from build123d import *

# Parameters (mm, degrees)
SKETCH5_R                   = 7.5
CUT_EXTRUDE1_DEPTH          = 90
SKETCH6_R                   = 3.5
CUT_EXTRUDE2_DEPTH          = 20
CIRPATTERN1_COUNT           = 6
SKETCH11_R                  = 3.18
CUT_EXTRUDE4_DEPTH          = 101.105860558
SKETCH23_R                  = 30.48
CUT_EXTRUDE6_DEPTH          = 80.122584091
F_1_4_CLEARANCE_HOLE1_D     = 6.5278
F_1_4_CLEARANCE_HOLE1_DEPTH = 15.4203
F_1_4_CLEARANCE_HOLE1_TIP   = 1.961148974
CHAMFER1_SIZE               = 3.175


with BuildPart() as part:
    # Sketch1 → Revolve1 (revolve)
    with BuildSketch(Plane(origin=(0, 0, 0), x_dir=(0, 0, -1), z_dir=(1, 0, 0))):
        Polygon((0, 30.35), (12.7, 30.35), (12.7, 6.35), (30.48, 6.35), (30.48, 0), (15.68, 0), (10.16, -20.600920458), (10.16, -60), (0, -60), align=None)
    revolve(axis=Axis((0, 0, 0), (0, 1, 0)))

    # Sketch5 → Cut-Extrude1 (cut)
    with BuildSketch(Plane.XZ.offset(60)):
        with Locations(Location((0, 0, 0), (0, 0, 270))):
            Circle(SKETCH5_R)
    extrude(amount=-CUT_EXTRUDE1_DEPTH, mode=Mode.SUBTRACT)

    # Sketch6 → Cut-Extrude2 (cut, symmetric)
    with BuildSketch(Plane.XY):
        with Locations((0, 16.659966967)):
            Circle(SKETCH6_R)
    cut_extrude2 = extrude(amount=CUT_EXTRUDE2_DEPTH, both=True, mode=Mode.SUBTRACT)

    # CirPattern1: Cut-Extrude2 ×6 about axis
    cirpattern1_axis = Axis((0, 30.35, 0), (0, -1, 0))
    for i in range(1, CIRPATTERN1_COUNT):
        add(cut_extrude2.rotate(cirpattern1_axis, i * 360 / CIRPATTERN1_COUNT), mode=Mode.SUBTRACT)

    # Sketch11 → Cut-Extrude4 (cut, through all)
    with BuildSketch(Plane(origin=(0, 30.35, 0), x_dir=(1, 0, 0), z_dir=(0, 1, 0))):
        with Locations(Location((0, 0, 0), (0, 0, 270))):
            Circle(SKETCH11_R)
    extrude(amount=-CUT_EXTRUDE4_DEPTH, mode=Mode.SUBTRACT)

    # Sketch23 → Cut-Extrude6 (cut, through all)
    with BuildSketch(Plane(origin=(0, 6.35, 0), x_dir=(1, 0, 0), z_dir=(0, 1, 0))):
        with Locations(Location((0, 0, 0), (0, 0, 90))):
            Circle(SKETCH23_R)
    extrude(amount=CUT_EXTRUDE6_DEPTH, mode=Mode.SUBTRACT)

    # 1_4 Clearance Hole1
    with Locations(Plane(origin=(0, 6.35, 0), x_dir=(1, 0, 0), z_dir=(0, 1, 0))):
        with Locations((3.330049479, 25.294237026), (-20.240427094, 15.531025958), (23.570476573, 9.763211068), (20.240427094, -15.531025958), (-3.330049479, -25.294237026), (-23.570476573, -9.763211068)):
            Hole(F_1_4_CLEARANCE_HOLE1_D / 2, depth=F_1_4_CLEARANCE_HOLE1_DEPTH)
            with Locations((0, 0, -(F_1_4_CLEARANCE_HOLE1_DEPTH + F_1_4_CLEARANCE_HOLE1_TIP / 2))):  # 118° drill point
                Cone(0, F_1_4_CLEARANCE_HOLE1_D / 2, F_1_4_CLEARANCE_HOLE1_TIP, mode=Mode.SUBTRACT)

    # Chamfer1
    chamfer1_edges = [part.edges().sort_by_distance(p)[0] for p in [
        (0, 6.35, 7.5),
    ]]
    chamfer(chamfer1_edges, length=CHAMFER1_SIZE)


solid = part.part
Part model, mm, in its own coordinate system. A direction names the side the tool comes from. Give positions to 0.01 mm unless a question says otherwise; leave off trailing zeros. Loops run counter-clockwise (first coordinate to the right, second up) from the corner with the lowest first, then second, coordinate; pieces in that order, holes last. Notation, with made-up numbers: M -33,-21.75 L -6,-21.75 A24 ccw -6,5.25 Z; hole C 84.25,-38.75 d11. An arc over 180 degrees is marked long. Put each result on its own line as item: value. Start each with the question number.
1) Flat gauge pins, fed straight in: pin 1 (5 mm diameter, centred on y = -5.5, z = 2, fed in from +X); pin 2 (1 mm diameter, centred on y = -46, z = 3, fed in from -X); pin 3 (10 mm diameter, centred on x = -1, y = -33, fed in from +Z); pin 4 (5 mm diameter, centred on x = -20.24, z = -15.53, fed in from +Y). Where does each tip first touch, or does it go through?
2) Saw through at C-C (z = -23.5). List the corners of the cut face in (x, y), then the cut area to 3 significant figures.
3) Saw through at B-B (y = -30). List the corners of the cut face in (x, z), then the cut area to 3 significant figures.
4) Probe probe 1 along Y at (x, z) = (27, -3); probe 2 along X at (y, z) = (-5, 3); probe 3 along Z at (x, y) = (-2.5, -42.5). List the from-to ranges inside material, lowest first.
5) Pull direction Z, two halves, no side cores. Call faces 1 (the conical face through (11.976, -12.734, 2.659)), 2 (the flat face through (6, -60, 5)), 3 (the cylindrical face through (17.127, 3.131, 14.551)): +Z half, -Z half, draft (parallel to the pull), parting line (faces both ways), or undercut.
6) 3-axis set-ups, long thin cutter, end or side, ignore diameter. For faces 4 (the cylindrical face through (-26.684, 3.131, 8.783)), 5 (the cylindrical face through (-10.074, -40.576, 1.323)): which of +Z, -Z, +X, -X, +Y, -Y reach the whole face in a straight line?
7) Saw through at D-D (x = -3). State how many separate pieces and enclosed holes the cut face has, then the cut area to 3 significant figures.
8) Saw through at A-A (z = 0). List the corners of the cut face in (x, y) (3 decimals).
Numbers:
1. pin 1: x = 14.79
1. pin 2: x = -9.85
1. pin 3: z = 10.16
1. pin 4: through
2. outline: M -19.41,0 L 0.6,0 L 0.6,6.35 L -19.41,6.35 Z; M 6.06,0 L 19.41,0 L 19.41,6.35 L 6.06,6.35 Z
2. area: 212 mm^2
3. outline: C 0,0 d20.32; hole C 0,0 d15
3. area: 148 mm^2
4. probe 1: 0 to 6.35
4. probe 2: -14.02 to -6.87, 6.87 to 14.02
4. probe 3: -9.85 to -7.07, 7.07 to 9.85
5. face 1: parting line
5. face 2: draft
5. face 3: undercut
6. face 4: +Y, -Y
6. face 5: -Y
7. separate pieces: 3
7. enclosed holes: 0
7. area: 703 mm^2
8. outline: M -30.48,0 L -15.68,0 L -10.16,-20.601 L -10.16,-60 L -7.5,-60 L -7.5,3.175 L -10.675,6.35 L -30.48,6.35 Z; M 7.5,-60 L 10.16,-60 L 10.16,-20.601 L 15.68,0 L 30.48,0 L 30.48,6.35 L 10.675,6.35 L 7.5,3.175 Z
